Check sheet for the modelled part. Datum: model origin and axes. Units: mm. A direction names the side the tool comes from. Give positions to 0.01 mm unless a question says otherwise; leave off trailing zeros. Loops run counter-clockwise (first coordinate to the right, second up) from the corner with the lowest first, then second, coordinate; pieces in that order, holes last. Notation, with made-up numbers: (82.5, 5) - (128.5, 5) arc R36 cw to (128.5, 41) - close; hole circle Ø2 at (-32, 38.5). An arc over 180 degrees is marked (long way). Use CSV: the item, a comma, the result in double quotes.
from build123d import *

# Parameters (mm, degrees)
SKETCH1_W           = 200
SKETCH1_H           = 160
BOSS_EXTRUDE3_DEPTH = 10
SKETCH3_R           = 5.25
SKETCH3_W           = 160
SKETCH3_H           = 120
CUT_EXTRUDE2_DEPTH  = 5
SKETCH6_R           = 5.25
CUT_EXTRUDE4_DEPTH  = 129.16005618


with BuildPart() as part:
    # Sketch1 → Boss-Extrude3 (new body)
    with BuildSketch(Plane(origin=(0, 0, 0), x_dir=(1, 0, 0), z_dir=(0, 1, 0))):
        Rectangle(SKETCH1_W, SKETCH1_H)
    extrude(amount=BOSS_EXTRUDE3_DEPTH)

    # Sketch3 → Cut-Extrude2 (cut)
    with BuildSketch(Plane(origin=(0, 10, 0), x_dir=(1, 0, 0), z_dir=(0, 1, 0))):
        with Locations(Location((-90, 70, 0), (0, 0, 270))):
            Circle(SKETCH3_R)
        with Locations(Location((90, -70, 0), (0, 0, 270))):
            Circle(SKETCH3_R)
        with Locations(Location((90, 70, 0), (0, 0, 270))):
            Circle(SKETCH3_R)
        with Locations(Location((-90, -70, 0), (0, 0, 270))):
            Circle(SKETCH3_R)
        Rectangle(SKETCH3_W, SKETCH3_H)
    extrude(amount=-CUT_EXTRUDE2_DEPTH, mode=Mode.SUBTRACT)

    # Sketch6 → Cut-Extrude4 (cut, through all)
    with BuildSketch(Plane(origin=(0, 5, 0), x_dir=(1, 0, 0), z_dir=(0, 1, 0))):
        with Locations(Location((-90, 70, 0), (0, 0, 270))):
            Circle(SKETCH6_R)
        with Locations(Location((90, 70, 0), (0, 0, 270))):
            Circle(SKETCH6_R)
        with Locations(Location((90, -70, 0), (0, 0, 270))):
            Circle(SKETCH6_R)
        with Locations(Location((-90, -70, 0), (0, 0, 270))):
            Circle(SKETCH6_R)
    extrude(amount=-CUT_EXTRUDE4_DEPTH, mode=Mode.SUBTRACT)


solid = part.part
1. Release check for a two-part mould opening along X. For faces 1 (the face through (-1, 8, -60)), 2 (the face through (100, 5, 1)), 3 (the face through (-1, 0, -1)), 4 (the face through (-1, 5, -1)) record: released by +X, released by -X, zero draft, split by the parting line, or undercut.
Completed:
face 1,"undercut"
face 2,"released by +X"
face 3,"zero draft"
face 4,"undercut"
2. Sectioned sample at D-D, the plane z = -39.5. Record the boundary of the cut face in (x, y), and give its area (3 significant figures).
Completed:
outline,"(-100, 0) - (100, 0) - (100, 10) - (80, 10) - (80, 5) - (-80, 5) - (-80, 10) - (-100, 10) - close"
area,"1,200 mm²"
3. Sectioned sample at A-A, the plane z = 70. Record the boundary of the cut face in (x, y).
Completed:
outline,"(-100, 0) - (-95.25, 0) - (-95.25, 10) - (-100, 10) - close; (-84.75, 0) - (84.75, 0) - (84.75, 10) - (-84.75, 10) - close; (95.25, 0) - (100, 0) - (100, 10) - (95.25, 10) - close"
4. Sectioned sample at C-C, the plane x = -15. Record the boundary of the cut face in (y, z), and give its area (3 significant figures).
Completed:
outline,"(0, -80) - (10, -80) - (10, -60) - (5, -60) - (5, 60) - (10, 60) - (10, 80) - (0, 80) - close"
area,"1,000 mm²"
5. Go/stop test with flat-tipped pins: pin 1 Ø6.5 at (x, z) = (-90, 70) entering from -Y; pin 2 Ø2 at (x, z) = (-18, 58.5) entering from +Y. Record where each tip stops, or that it passes through.
Completed:
pin 1,"passes through"
pin 2,"stops at y = 5"
6. Sectioned sample at B-B, the plane x = -90. Record the boundary of the cut face in (y, z), and give its area (3 significant figures).
Completed:
outline,"(0, -80) - (10, -80) - (10, -75.25) - (0, -75.25) - close; (0, -64.75) - (10, -64.75) - (10, 64.75) - (0, 64.75) - close; (0, 75.25) - (10, 75.25) - (10, 80) - (0, 80) - close"
area,"1,390 mm²"
7. Set-up check for faces 5 (the face through (80, 8, 1)), 6 (the face through (-89.769, 5.07, -75.245)): record each of +Z, -Z, +X, -X, +Y, -Y from which the full face is reachable in a straight line by a thin tool's end or side.
Completed:
face 5,"+Y"
face 6,"+Y, -Y"
8. Scan lines: line 1 along X through (y, z) = (3, -70); line 2 along Z through (x, y) = (2, 6.5); line 3 along X through (y, z) = (7.75, -2). Record each from-to range of solid material in increasing order.
Completed:
line 1,"x = -100 to -95.25, -84.75 to 84.75, 95.25 to 100"
line 2,"z = -80 to -60, 60 to 80"
line 3,"x = -100 to -80, 80 to 100"
